from build123d import *


with BuildPart() as part:
    # Sketch1 → Revolve1 (revolve)
    with BuildSketch(Plane.XY):
        Polygon((-13.146540644, 2.5), (-18.75, 2.5), (-18.75, 2), (-17.75, 2), (-17.75, 0), (-1.5, 0), (-1.5, 2.5), align=None)
    revolve1 = revolve(axis=Axis((0, 14.394370017, 0), (0, -1, 0)))

    # Mirror1: Revolve1 across Top Plane
    add(revolve1.mirror(Plane(origin=(0, 0, 0), x_dir=(1, 0, 0), z_dir=(0, 1, 0))))


solid = part.part
The listing builds one solid part. Answer for the finished solid, in the listing's coordinates (mm). A direction names the side the tool comes from. Give positions to 0.01 mm unless a question says otherwise; leave off trailing zeros. Order: outer loops, then holes, each group sorted by start corner. A loop starts at its lowest first (then second) coordinate and runs counter-clockwise, first axis right, second up. Notation, with made-up numbers: (61, 74.5) -> (102, 74.5) arc R16 cw to (102, 82.5) -> close; hole circle Ø1 at (39.5, 85). An arc over 180 degrees is marked (long way). Put each result on its own line as item: value.
Item 1: A cutting plane is placed at B-B on x = 0. Give the vertices of the cut face in (y, z).
Established:
outline: (-2.5, -18.75) -> (-2, -18.75) -> (-2, -17.75) -> (2, -17.75) -> (2, -18.75) -> (2.5, -18.75) -> (2.5, -1.5) -> (-2.5, -1.5) -> close; (-2.5, 1.5) -> (2.5, 1.5) -> (2.5, 18.75) -> (2, 18.75) -> (2, 17.75) -> (-2, 17.75) -> (-2, 18.75) -> (-2.5, 18.75) -> close
Item 2: A cutting plane is placed at C-C on z = 15.5. Give the vertices of the cut face in (x, y).
Established:
outline: (-10.55, -2.5) -> (10.55, -2.5) -> (10.55, -2) -> (8.65, -2) -> (8.65, 2) -> (10.55, 2) -> (10.55, 2.5) -> (-10.55, 2.5) -> (-10.55, 2) -> (-8.65, 2) -> (-8.65, -2) -> (-10.55, -2) -> close
Item 3: Straight lines are drawn through the part: line 1 (Z direction, x = 0, y = -0.15); line 2 (X direction, y = 0.25, z = 7). For each, find the intervals that lie inside material, in ascending order.
Established:
line 1: z = -17.75 to -1.5, 1.5 to 17.75
line 2: x = -16.31 to 16.31
Item 4: For faces 1 (the face through (-17, -2, 7)), 2 (the face through (0, -2.5, 4)), determine the directions among +Z, -Z, +X, -X, +Y, -Y from which every point of the face is accessible in a straight line to the end or side of a thin tool.
Established:
face 1: none
face 2: +Z, -Z, +X, -X, -Y
Item 5: A cutting plane is placed at A-A on z = 0. Give the vertices of the cut face in (x, y).
Established:
outline: (-18.75, -2.5) -> (-1.5, -2.5) -> (-1.5, 2.5) -> (-18.75, 2.5) -> (-18.75, 2) -> (-17.75, 2) -> (-17.75, -2) -> (-18.75, -2) -> close; (1.5, -2.5) -> (18.75, -2.5) -> (18.75, -2) -> (17.75, -2) -> (17.75, 2) -> (18.75, 2) -> (18.75, 2.5) -> (1.5, 2.5) -> close
Item 6: Given P1, Ø5, axis at x = 0, z = 0, coming from the -Y side; P2, Ø3, axis at y = 1.5, z = 2.5, coming from the -X side; P3, Ø1.5, axis at y = -2, z = 13.5, coming from the -X side, each flat-ended and moving along its own axis, determine where each tip first touches the part or whether it passes through.
Established:
P1: stops at y = -2.5
P2: stops at x = -18.72
P3: stops at x = -13.75
Item 7: A cutting plane is placed at D-D on x = 6. Give the vertices of the cut face in (y, z), plus the area to 3 significant figures.
Established:
outline: (-2.5, -17.76) -> (-2, -17.76) -> (-2, -16.71) -> (2, -16.71) -> (2, -17.76) -> (2.5, -17.76) -> (2.5, 17.76) -> (2, 17.76) -> (2, 16.71) -> (-2, 16.71) -> (-2, 17.76) -> (-2.5, 17.76) -> close
area: 169 mm^2
Item 8: For a pull along Z with two mould halves and no side action, classify faces 3 (the face through (2.44, 2.25, -18.59)), 4 (the face through (-17, 2, 7)), 5 (the face through (1.5, -0.04, -0.07)) as released by +Z, released by -Z, zero draft, split by the parting line, or undercut.
Established:
face 3: split by the parting line
face 4: zero draft
face 5: undercut
